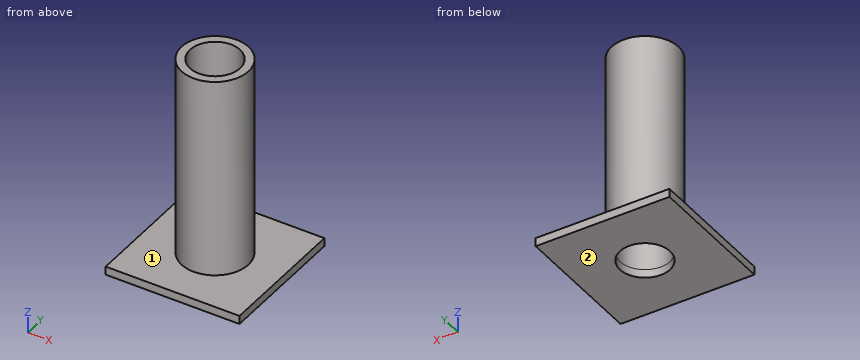
from build123d import *

# Parameters (mm, degrees)
F0_R     = 12.7
F0_R_2   = 9.525
F1_DEPTH = 76.2
F2_W     = 50.8
F2_H     = 50.8
F2_R     = 9.525
F3_DEPTH = 3.175


with BuildPart() as f1:
    # F0 (on Top) → F1 (new body)
    with BuildSketch(Plane.XY):
        Circle(F0_R)
        Circle(F0_R_2, mode=Mode.SUBTRACT)
    extrude(amount=F1_DEPTH)

    # F2 (on Top) → F3 (join)
    with BuildSketch(Plane.XY):
        Rectangle(F2_W, F2_H)
        Circle(F2_R, mode=Mode.SUBTRACT)
    extrude(amount=-F3_DEPTH)


solid = f1.part
Read the model definition and answer for the solid it produces. Units are mm, in the model's axes. Face numbers are marked on the shaded views. A direction names the side the tool comes from. Give positions to 0.01 mm unless a question says otherwise; leave off trailing zeros. Write each loop counter-clockwise with the first axis right and the second up, starting at its lowest first coordinate (ties: lowest second). Pieces come first, ordered by that corner, then holes. Notation, with made-up numbers: (26, 63.5) - (49, 63.5) arc R10 cw to (49, 72.5) - close; hole circle Ø3 at (-21, 16.25). An arc over 180 degrees is marked (long way). Answer in a Markdown table with one row per item. Add a question column.
Item 1: Section D-D, the plane x = 11 is taken. Write down the section's boundary in (y, z) (3 decimals), and give its area (3 significant figures).
Item 2: Section C-C, the plane z = 59 is taken. Write down the section's boundary in (x, y) (3 decimals).
Item 3: A tool of negligible diameter and unlimited length cuts with its end or side. For the marked faces 1 and 2, from which of +Z, -Z, +X, -X, +Y, -Y can it reach the whole face along a straight path? Write none if from no direction.
Item 4: Section A-A, the plane y = 0 is taken. Write down the section's boundary in (x, z) (3 decimals), and give its area (3 significant figures).
Item 5: Find the intervals of material crossed by L1, parallel to Y at x = 0, z = -1.35 (3 decimals); L2, parallel to Y at x = 0, z = 16.5 (3 decimals); L3, parallel to Z at x = -8, y = -22 (3 decimals), in increasing order.
Item 6: Flat-ended cylindrical pins translate along their axes: P1, Ø5, axis at x = -8, z = 5.5, coming from the +Y side; P2, Ø12, axis at x = 1.5, z = 57, coming from the +Y side; P3, Ø4, axis at x = -11, z = 59, coming from the +Y side. Find the tip coordinate at first contact, or state that the pin passes through.
Recorded:
| question | item | result |
|---|---|---|
| 1 | outline | (-25.4, -3.175) - (25.4, -3.175) - (25.4, 0) - (6.347, 0) - (6.347, 76.2) - (-6.347, 76.2) - (-6.347, 0) - (-25.4, 0) - close |
| 1 | area | 1,130 mm2 |
| 2 | outline | circle Ø25.4 at (0, 0); hole circle Ø19.05 at (0, 0) |
| 3 | face 1 | +Z |
| 3 | face 2 | -Z, +X, -X, +Y, -Y |
| 4 | outline | (-25.4, -3.175) - (-9.525, -3.175) - (-9.525, 76.2) - (-12.7, 76.2) - (-12.7, 0) - (-25.4, 0) - close; (9.525, -3.175) - (25.4, -3.175) - (25.4, 0) - (12.7, 0) - (12.7, 76.2) - (9.525, 76.2) - close |
| 4 | area | 585 mm2 |
| 5 | L1 | y = -25.4 to -9.525, 9.525 to 25.4 |
| 5 | L2 | y = -12.7 to -9.525, 9.525 to 12.7 |
| 5 | L3 | z = -3.175 to 0 |
| 6 | P1 | stops at y = 11.45 |
| 6 | P2 | stops at y = 12.7 |
| 6 | P3 | stops at y = 8.96 |
